Design review of the part built by this model. Coordinates are the model's own, in mm. Face numbers are marked on the shaded views. A direction names the side the tool comes from. Round coordinates to 2 decimals unless told otherwise and drop trailing zeros. Order: outer loops, then holes, each group sorted by start corner. A loop starts at its lowest first (then second) coordinate and runs counter-clockwise, first axis right, second up. Notation, with made-up numbers: (8.25, 77.5) - (49.25, 77.5) arc R30 cw to (49.25, 115.5) - close; hole circle Ø11 at (63, 16.25). An arc over 180 degrees is marked (long way). Write item = value, one per line.
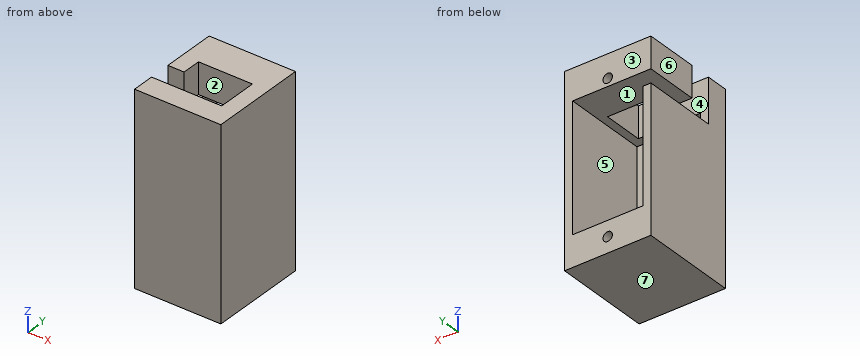
from build123d import *

# Parameters (mm, degrees)
SKETCH1_W           = 16
SKETCH1_H           = 35
BOSS_EXTRUDE1_DEPTH = 18.2
SKETCH2_W           = 13
SKETCH2_H           = 23.5
CUT_EXTRUDE1_DEPTH  = 15.7
SKETCH3_R           = 0.875
CUT_EXTRUDE2_DEPTH  = 5
SKETCH4_W           = 10
SKETCH4_H           = 7.5
CUT_EXTRUDE3_DEPTH  = 5.75
SKETCH5_W           = 2.5
SKETCH5_H           = 12.5
CUT_EXTRUDE4_DEPTH  = 1.5
SKETCH6_W           = 8.25
SKETCH6_H           = 4
CUT_EXTRUDE5_DEPTH  = 3


with BuildPart() as part:
    # Sketch1 → Boss-Extrude1 (new body)
    with BuildSketch(Plane(origin=(0, 0, 0), x_dir=(1, 0, 0), z_dir=(0, 1, 0))):
        Rectangle(SKETCH1_W, SKETCH1_H)
    extrude(amount=BOSS_EXTRUDE1_DEPTH)

    # Sketch2 → Cut-Extrude1 (cut)
    with BuildSketch(Plane(origin=(0, 18.2, 0), x_dir=(1, 0, 0), z_dir=(0, 1, 0))):
        Rectangle(SKETCH2_W, SKETCH2_H)
    extrude(amount=-CUT_EXTRUDE1_DEPTH, mode=Mode.SUBTRACT)

    # Sketch3 → Cut-Extrude2 (cut)
    with BuildSketch(Plane(origin=(0, 18.2, 0), x_dir=(1, 0, 0), z_dir=(0, 1, 0))):
        with Locations(Location((0, -13.2, 0), (0, 0, 270))):
            Circle(SKETCH3_R)
        with Locations(Location((0, 14.6, 0), (0, 0, 270))):
            Circle(SKETCH3_R)
    extrude(amount=-CUT_EXTRUDE2_DEPTH, mode=Mode.SUBTRACT)

    # Sketch4 → Cut-Extrude3 (cut)
    with BuildSketch(Plane(origin=(0, 0, 11.75), x_dir=(-1, 0, 0), z_dir=(0, 0, -1))):
        with Locations((0, 7.9)):
            Rectangle(SKETCH4_W, SKETCH4_H)
    extrude(amount=-CUT_EXTRUDE3_DEPTH, mode=Mode.SUBTRACT)

    # Sketch5 → Cut-Extrude4 (cut)
    with BuildSketch(Plane.ZY.offset(8)):
        with Locations((10.5, 11.95)):
            Rectangle(SKETCH5_W, SKETCH5_H)
    extrude(amount=-CUT_EXTRUDE4_DEPTH, mode=Mode.SUBTRACT)

    # Sketch6 → Cut-Extrude5 (cut)
    with BuildSketch(Plane.ZY.offset(8)):
        with Locations((13.375, 6.15)):
            Rectangle(SKETCH6_W, SKETCH6_H)
    extrude(amount=-CUT_EXTRUDE5_DEPTH, mode=Mode.SUBTRACT)


solid = part.part
Item 1: For the marked faces 1, 2, 3 and 4, list the 3-axis set-ups (+Z, -Z, +X, -X, +Y, -Y) from which the entire face can be reached by the end or side of a thin tool; tool diameter is ignored.
Data:
face_1 = +Y
face_2 = +Z
face_3 = +Z, -Z, +X, -X, +Y
face_4 = +Z, -X
Item 2: The part is to be moulded in two halves that separate along Z. For the marked faces 5, 6 and 7, say which applies: +Z half, -Z half, draft (parallel to the pull), parting line (faces both ways), or undercut.
Data:
face_5 = undercut
face_6 = draft
face_7 = -Z half
Item 3: Take a section at A-A, the plane x = 0. State the section outline as (y, z) points (3 decimals).
Data:
outline = (0, -17.5) - (18.2, -17.5) - (18.2, -15.475) - (13.2, -15.475) - (13.2, -13.725) - (18.2, -13.725) - (18.2, -11.75) - (2.5, -11.75) - (2.5, 11.75) - (4.15, 11.75) - (4.15, 17.5) - (0, 17.5) - close; (11.65, 11.75) - (18.2, 11.75) - (18.2, 12.325) - (13.2, 12.325) - (13.2, 14.075) - (18.2, 14.075) - (18.2, 17.5) - (11.65, 17.5) - close
Item 4: Take a section at C-C, the plane x = 2. State the section outline as (y, z) points, and give its area (3 significant figures).
Data:
outline = (0, -17.5) - (18.2, -17.5) - (18.2, -11.75) - (2.5, -11.75) - (2.5, 11.75) - (4.15, 11.75) - (4.15, 17.5) - (0, 17.5) - close; (11.65, 11.75) - (18.2, 11.75) - (18.2, 17.5) - (11.65, 17.5) - close
area = 225 mm2
Item 5: Insertion check: P1, Ø4, axis at x = -3, z = 0.5, coming from the +Y side; P2, Ø0.5, axis at x = 0, z = 13, coming from the +Y side; P3, Ø4, axis at x = 1.5, y = 7.5, coming from the +Z side. Each pin has a flat end and moves straight along its axis. Give the tip position at first contact, or say it passes through.
Data:
P1 = 2.5
P2 = 13.2
P3 = -11.75
Item 6: For line 1 along X through (y, z) = (16.55, -14.6) (3 decimals); line 2 along X through (y, z) = (5, -8); line 3 along Z through (x, y) = (-7.5, 16.25), list the stretches that pass through material, from the lowest coordinate up. Write a range as [from, to].
Data:
line_1 = [-8, -0.875], [0.875, 8]
line_2 = [-8, -6.5], [6.5, 8]
line_3 = [-17.5, 9.25], [11.75, 17.5]
Item 7: Take a section at D-D, the plane z = -14.6. State the section outline as (x, y) points (3 decimals), and give its area (3 significant figures).
Data:
outline = (-8, 0) - (8, 0) - (8, 18.2) - (0.875, 18.2) - (0.875, 13.2) - (-0.875, 13.2) - (-0.875, 18.2) - (-8, 18.2) - close
area = 282 mm2
Item 8: Take a section at B-B, the plane y = 17. State the section outline as (x, z) points (3 decimals), and give its area (3 significant figures).
Data:
outline = (-8, -17.5) - (8, -17.5) - (8, 17.5) - (-8, 17.5) - (-8, 11.75) - (6.5, 11.75) - (6.5, -11.75) - (-6.5, -11.75) - (-6.5, 9.25) - (-8, 9.25) - close; hole circle Ø1.75 at (0, -14.6); hole circle Ø1.75 at (0, 13.2)
area = 246 mm2
